Design review of the part built by this model. Coordinates are the model's own, in mm. Face numbers are marked on the shaded views. Give positions to 0.01 mm unless a question says otherwise; leave off trailing zeros. Loops run counter-clockwise (first coordinate to the right, second up) from the corner with the lowest first, then second, coordinate; pieces in that order, holes last. Notation, with made-up numbers: (51.5, 24.5) -> (71.5, 24.5) arc R12 cw to (71.5, 34.5) -> close; hole circle Ø7 at (66.5, 56). An arc over 180 degrees is marked (long way). Use a Markdown table: item, result. Add a question column.
1. Add section A-A (z = 15.5). State the section outline as (x, y) points.
2. Add section C-C (y = 0). Count the separate pieces of the cut face and the enclosed holes in it, and give its area (3 significant figures).
3. For pin 1 Ø7 at (y, z) = (9, 28) entering from +X; pin 2 Ø11 at (y, z) = (2, 44) entering from -X; pin 3 Ø3 at (x, y) = (0, -0.5) entering from +Z, all flat-tipped, find the tip position at first contact; note any pin that passes through.
4. Add section B-B (x = 0). State the section outline as (y, z) points, and give its area (3 significant figures).
5. Draft analysis for pull direction Z (two halves, no side actions). For the marked faces 1, 2, 3 and 4, state which applies: pulls with the +Z half, pulls with the -Z half, needs draft (parallel to the pull), parting line crosses it, or undercut.
6. Add section D-D (y = 12.25). State the section outline as (x, z) points.
7. To check wall thickness, follow line 1 (Y direction, x = -15, z = 2.5); line 2 (X direction, y = -6, z = 39.5); line 3 (X direction, y = 0, z = 13). State the ranges of each line that lie inside material, in increasing order.
```python
from build123d import *

# Parameters (mm, degrees)
ESQUISSE1_W                                          = 40
ESQUISSE1_H                                          = 30
BOSS_EXTRU_1_DEPTH                                   = 5
ESQUISSE5_W                                          = 50
ESQUISSE5_H                                          = 30
BOSS_EXTRU_3_DEPTH                                   = 30
ENL_V_MAT_EXTRU_1_DEPTH                              = 25
CHAMBRAGE_POUR_T_TE_CYLINDRIQUE_FENDUE_M_D           = 2.7
CHAMBRAGE_POUR_T_TE_CYLINDRIQUE_FENDUE_M_DEPTH       = 7
CHAMBRAGE_POUR_T_TE_CYLINDRIQUE_FENDUE_M_CBORE_D     = 5.5
CHAMBRAGE_POUR_T_TE_CYLINDRIQUE_FENDUE_M_CBORE_DEPTH = 1.8
CHAMBRAGE_POUR_T_TE_CYLINDRIQUE_FENDUE_M_TIP         = 0.811161836
ESQUISSE14_W                                         = 3
ESQUISSE14_H                                         = 8
ENL_V_MAT_EXTRU_2_DEPTH                              = 61.415229868
D_GAGEMENT_M31_D                                     = 3.2
D_GAGEMENT_M31_DEPTH                                 = 7
D_GAGEMENT_M31_TIP                                   = 0.96137699
ESQUISSE16_W                                         = 50
ESQUISSE16_H                                         = 30
ESQUISSE16_R                                         = 3.5
BOSS_EXTRU_4_DEPTH                                   = 5
CONG_1_R                                             = 2
ESQUISSE17_W                                         = 10
ESQUISSE17_H                                         = 10
ENL_V_MAT_EXTRU_3_DEPTH                              = 2
BOSS_EXTRU_5_START                                   = 2
ESQUISSE18_R                                         = 6
ESQUISSE18_R_2                                       = 3.5
BOSS_EXTRU_5_DEPTH                                   = 2


with BuildPart() as part:
    # Esquisse1 → Boss.-Extru.1 (new body)
    with BuildSketch(Plane.XY):
        Rectangle(ESQUISSE1_W, ESQUISSE1_H)
    extrude(amount=BOSS_EXTRU_1_DEPTH)

    # Esquisse5 → Boss.-Extru.3 (add)
    with BuildSketch(Plane.ZY.offset(20)):
        with Locations((30, 0)):
            Rectangle(ESQUISSE5_W, ESQUISSE5_H)
    extrude(amount=-BOSS_EXTRU_3_DEPTH)

    # Esquisse6 → Enlèv. mat.-Extru.1 (cut)
    with BuildSketch(Plane.ZY.offset(20)):
        Polygon((50, 11), (50, 4), (55, 4), (55, -4), (50, -4), (50, -11), (5, -11), (5, 11), align=None)
    extrude(amount=-ENL_V_MAT_EXTRU_1_DEPTH, mode=Mode.SUBTRACT)

    # Chambrage pour tête cylindrique fendue M2.51
    with Locations(Plane.XY.offset(5)):
        with Locations((0, 0)):
            CounterBoreHole(CHAMBRAGE_POUR_T_TE_CYLINDRIQUE_FENDUE_M_D / 2, CHAMBRAGE_POUR_T_TE_CYLINDRIQUE_FENDUE_M_CBORE_D / 2, CHAMBRAGE_POUR_T_TE_CYLINDRIQUE_FENDUE_M_CBORE_DEPTH, depth=CHAMBRAGE_POUR_T_TE_CYLINDRIQUE_FENDUE_M_DEPTH)
            with Locations((0, 0, -(CHAMBRAGE_POUR_T_TE_CYLINDRIQUE_FENDUE_M_DEPTH + CHAMBRAGE_POUR_T_TE_CYLINDRIQUE_FENDUE_M_TIP / 2))):  # 118° drill point
                Cone(0, CHAMBRAGE_POUR_T_TE_CYLINDRIQUE_FENDUE_M_D / 2, CHAMBRAGE_POUR_T_TE_CYLINDRIQUE_FENDUE_M_TIP, mode=Mode.SUBTRACT)

    # Esquisse14 → Enlèv. mat.-Extru.2 (cut, through all)
    with BuildSketch(Plane.XY.offset(55)):
        with Locations((8.5, 0)):
            Rectangle(ESQUISSE14_W, ESQUISSE14_H)
    extrude(amount=-ENL_V_MAT_EXTRU_2_DEPTH, mode=Mode.SUBTRACT)

    # Dégagement M31
    with Locations(Plane.ZY.offset(20)):
        with Locations((2.5, -4), (2.5, 4)):
            Hole(D_GAGEMENT_M31_D / 2, depth=D_GAGEMENT_M31_DEPTH)
            with Locations((0, 0, -(D_GAGEMENT_M31_DEPTH + D_GAGEMENT_M31_TIP / 2))):  # 118° drill point
                Cone(0, D_GAGEMENT_M31_D / 2, D_GAGEMENT_M31_TIP, mode=Mode.SUBTRACT)

    # Esquisse16 → Boss.-Extru.4 (add)
    with BuildSketch(Plane(origin=(20, 0, 0), x_dir=(0, 0, -1), z_dir=(1, 0, 0))):
        with Locations((-30, 0)):
            Rectangle(ESQUISSE16_W, ESQUISSE16_H)
        with Locations((-43, 0)):
            Circle(ESQUISSE16_R, mode=Mode.SUBTRACT)
    extrude(amount=-BOSS_EXTRU_4_DEPTH)

    # Congé1
    cong_1_edges = [part.edges().sort_by_distance(p)[0] for p in [
        (12.5, -15, 5),
        (10, 9.5, 5),
        (10, 15, 30),
        (10, -9.5, 55),
        (-5, 15, 55),
        (10, -15, 30),
        (-5, -15, 55),
        (-20, -9.5, 55),
        (-20, 9.5, 55),
        (10, -9.5, 5),
        (10, 9.5, 55),
        (20, -15, 27.5),
        (-20, -15, 27.5),
        (-20, 15, 27.5),
        (20, 15, 27.5),
        (12.5, 15, 5),
        (15, -15, 30),
        (15, 0, 55),
        (17.5, -15, 55),
        (15, 15, 30),
        (17.5, 15, 55),
        (15, 0, 5),
        (20, 0, 55),
    ]]
    fillet(cong_1_edges, radius=CONG_1_R)

    # Esquisse17 → Enlèv. mat.-Extru.3 (cut)
    with BuildSketch(Plane.ZY.offset(-15)):
        with Locations((43, 0)):
            Rectangle(ESQUISSE17_W, ESQUISSE17_H)
    extrude(amount=-ENL_V_MAT_EXTRU_3_DEPTH, mode=Mode.SUBTRACT)

    # Esquisse18 → Boss.-Extru.5 (add)
    with BuildSketch(Plane(origin=(20, 0, 0), x_dir=(0, 0, -1), z_dir=(1, 0, 0)).offset(BOSS_EXTRU_5_START)):
        with Locations(Location((-43, 0, 0), (0, 0, 180))):
            Circle(ESQUISSE18_R)
        with Locations((-43, 0)):
            Circle(ESQUISSE18_R_2, mode=Mode.SUBTRACT)
    extrude(amount=-BOSS_EXTRU_5_DEPTH)


solid = part.part
```
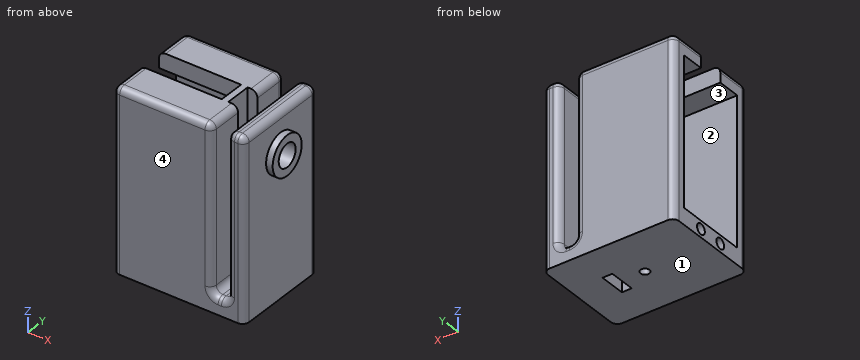
Taken from the geometry:
| question | item | result |
|---|---|---|
| 1 | outline | (-20, -13) arc R2 ccw to (-18, -15) -> (8, -15) arc R2 ccw to (10, -13) -> (10, -4) -> (7, -4) -> (7, 4) -> (10, 4) -> (10, 13) arc R2 ccw to (8, 15) -> (-18, 15) arc R2 ccw to (-20, 13) -> (-20, 11) -> (5, 11) -> (5, -11) -> (-20, -11) -> close; (15, -13) arc R2 ccw to (17, -15) -> (18, -15) arc R2 ccw to (20, -13) -> (20, 13) arc R2 ccw to (18, 15) -> (17, 15) arc R2 ccw to (15, 13) -> close |
| 2 | separate pieces | 4 |
| 2 | enclosed holes | 0 |
| 2 | area | 485 mm^2 |
| 3 | pin 1 | stops at x = 20 |
| 3 | pin 2 | stops at x = 5 |
| 3 | pin 3 | stops at z = 3.2 |
| 4 | outline | (-15, 0) -> (-1.35, 0) -> (-1.35, 3.2) -> (-2.75, 3.2) -> (-2.75, 5) -> (-11, 5) -> (-11, 50) -> (-4, 50) -> (-4, 55) -> (-13, 55) arc R2 ccw to (-15, 53) -> close; (1.35, 0) -> (15, 0) -> (15, 53) arc R2 ccw to (13, 55) -> (4, 55) -> (4, 50) -> (11, 50) -> (11, 5) -> (2.75, 5) -> (2.75, 3.2) -> (1.35, 3.2) -> close |
| 4 | area | 600 mm^2 |
| 5 | face 1 | pulls with the -Z half |
| 5 | face 2 | undercut |
| 5 | face 3 | undercut |
| 5 | face 4 | needs draft |
| 6 | outline | (-20, 0) -> (20, 0) -> (20, 53) arc R2 ccw to (18, 55) -> (17, 55) arc R2 ccw to (15, 53) -> (15, 7) arc R2 cw to (13, 5) -> (12, 5) arc R2 cw to (10, 7) -> (10, 53) arc R2 ccw to (8, 55) -> (-18, 55) arc R2 ccw to (-20, 53) -> close |
| 7 | line 1 | y = -15 to -5.6, -2.4 to 2.4, 5.6 to 15 |
| 7 | line 2 | x = 5 to 10, 15 to 20 |
| 7 | line 3 | x = 5 to 7, 15 to 20 |
